```python
from build123d import *

# Parameters (mm, degrees)
F1_DEPTH = 127
F2_T     = -2.54
F3_W     = 219.6087762713
F3_H     = 111.9595093346
F4_DEPTH = 114.3


with BuildPart() as f1:
    # F0 (on Front) → F1 (new body)
    with BuildSketch(Plane.XZ):
        Polygon((-9.013194183, 43.6832010746), (-153.9823263884, 43.6832010746), (-153.9823263884, -76.7388492823), (76.2072727084, -76.7388492823), (76.2072727084, -73.0584636331), (-135.6322020292, -73.0584636331), (-38.0154103041, 16.9434007257), align=None)
        Polygon((76.2072727084, 43.6832010746), (-9.013194183, 43.6832010746), (-38.0154103041, 16.9434007257), (76.2072727084, 16.9434007257), align=None)
        Polygon((76.2072727084, 16.9434007257), (-38.0154103041, 16.9434007257), (-135.6322020292, -73.0584636331), (76.2072727084, -73.0584636331), align=None)
    extrude(amount=F1_DEPTH)

    # F2
    f2_openings = [f1.faces().sort_by_distance(p)[0] for p in [
        (-38.887527, -127, -16.527824),
        (76.207273, -63.5, -16.527824),
    ]]
    offset(amount=F2_T, openings=f2_openings)

    # F3 (on face) → F4 (join)
    with BuildSketch(Plane.XZ.offset(2.54)):
        with Locations((-33.5971154273, -18.219094615)):
            Rectangle(F3_W, F3_H)
    extrude(amount=F4_DEPTH)


solid = f1.part
```
Work out the finished part from the listing and answer in its coordinate system (mm). A direction names the side the tool comes from. Coordinates: 2 decimals unless noted, no trailing zeros. Loops run counter-clockwise (first coordinate to the right, second up) from the corner with the lowest first, then second, coordinate; pieces in that order, holes last. Notation, with made-up numbers: (-10, -23.5) - (39, -23.5) arc R15 cw to (39, -5.5) - close; hole circle Ø10 at (-40, 86). An arc over 180 degrees is marked (long way). Use a Markdown table: item, result.
Item 1: For faces 4 (the flat face through (76.207, -48, -17)), 5 (the flat face through (-35, -116.84, -17)), 6 (the flat face through (-151.442, -64, -16)), determine the directions among +Z, -Z, +X, -X, +Y, -Y from which every point of the face is accessible in a straight line to the end or side of a thin tool.
Evaluation:
| item | result |
|---|---|
| face 4 | +Z, -Z, +X, +Y, -Y |
| face 5 | +X, -Y |
| face 6 | -Y |
Item 2: Consider probe 1 along Z at (x, y) = (47, -79.5); probe 2 along X at (y, z) = (-84, 11); probe 3 along Y at (x, z) = (-9, 39). Determine where each line is inside the solid, lowest interval first. Write a range as from..to.
Evaluation:
| item | result |
|---|---|
| probe 1 | z = -76.74..37.76, 41.14..43.68 |
| probe 2 | x = -153.98..-151.44, -143.4..76.21 |
| probe 3 | y = -2.54..0 |
Item 3: Given pin 1 Ø1 at (x, z) = (-27, -39.5) entering from -Y; pin 2 Ø4 at (x, z) = (14.5, 11) entering from +Y, each flat-ended and moving along its own axis, determine where each tip first touches the part or whether it passes through.
Evaluation:
| item | result |
|---|---|
| pin 1 | stops at y = -116.84 |
| pin 2 | stops at y = 0 |
Item 4: Find section C-C, the plane y = -88. Determine the outline of the cut face in (x, z).
Evaluation:
| item | result |
|---|---|
| outline | (-153.98, -76.74) - (76.21, -76.74) - (76.21, 37.76) - (-143.4, 37.76) - (-143.4, -74.2) - (-151.44, -74.2) - (-151.44, 41.14) - (76.21, 41.14) - (76.21, 43.68) - (-153.98, 43.68) - close |
Item 5: Find section B-B, the plane z = 6.5. Determine the outline of the cut face in (x, y).
Evaluation:
| item | result |
|---|---|
| outline | (-153.98, -127) - (-151.44, -127) - (-151.44, -2.54) - (-143.4, -2.54) - (-143.4, -116.84) - (76.21, -116.84) - (76.21, 0) - (-153.98, 0) - close |
Item 6: Find section A-A, the plane x = -133.5. Determine the outline of the cut face in (y, z), and give its area (3 significant figures).
Evaluation:
| item | result |
|---|---|
| outline | (-127, -76.74) - (0, -76.74) - (0, 43.68) - (-127, 43.68) - (-127, 41.14) - (-2.54, 41.14) - (-2.54, 37.76) - (-116.84, 37.76) - (-116.84, -74.2) - (-127, -74.2) - close |
| area | 13,700 mm2 |
Item 7: The mould has two halves that part along Z. Classify faces 1 (the flat face through (-40, 0, -16)), 2 (the flat face through (-37, -63, 43.683)), 3 (the flat face through (-143.402, -59, -19)): +Z half, -Z half, draft (parallel to the pull), parting line (faces both ways), or undercut.
Evaluation:
| item | result |
|---|---|
| face 1 | draft |
| face 2 | +Z half |
| face 3 | undercut |
